Geometry: see drawing. Coordinates: mm, zero at the bounding-box minimum. Coordinates: 2 decimals unless noted, no trailing zeros. Loops run counter-clockwise (first coordinate to the right, second up) from the corner with the lowest first, then second, coordinate; pieces in that order, holes last.
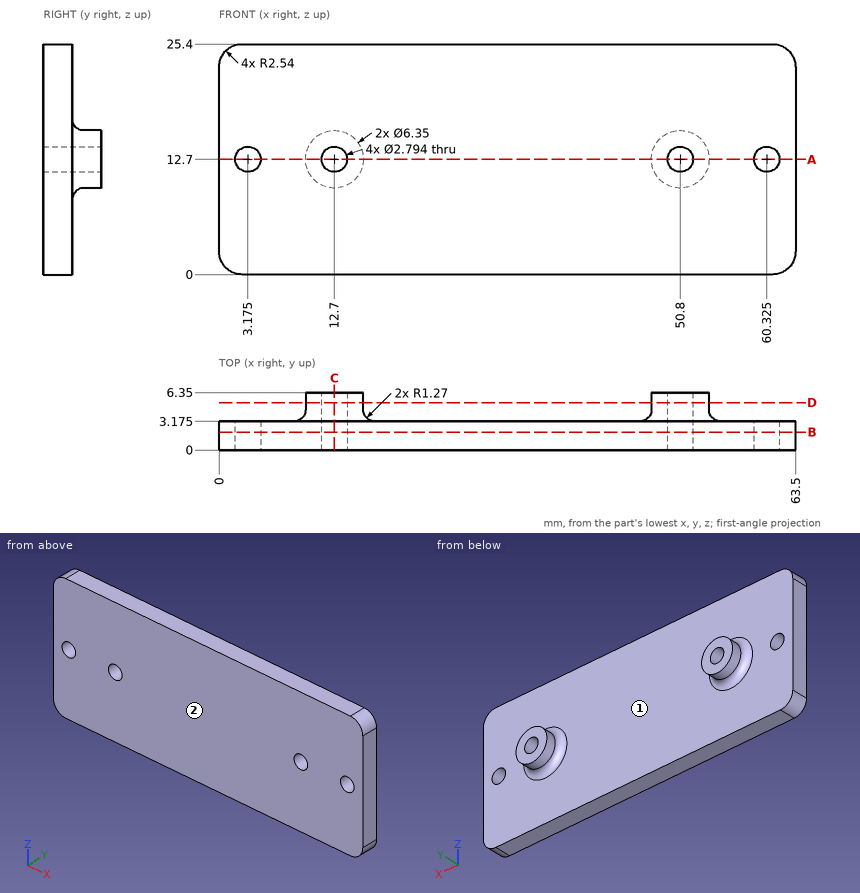
Item 1: Section query C-C (x = 12.7). Output: boundary loops of the cut face in (y, z) (3 decimals), then the cut area to 3 significant figures.
Result:
outline: (0, 0) - (3.175, 0) - (3.175, 8.255) arc R1.27 cw to (4.445, 9.525) - (6.35, 9.525) - (6.35, 11.303) - (0, 11.303) - close; (0, 14.097) - (6.35, 14.097) - (6.35, 15.875) - (4.445, 15.875) arc R1.27 cw to (3.175, 17.145) - (3.175, 25.4) - (0, 25.4) - close
area: 83.8 mm2
Item 2: Line query: L1, parallel to Z at x = 51, y = 1; L2, parallel to Z at x = 50.8, y = 5 (3 decimals); L3, parallel to Y at x = 31, z = 12 (3 decimals). Output: solid intervals per line, ascending.
Result:
L1: z = 0 to 11.32, 14.08 to 25.4
L2: z = 9.525 to 11.303, 14.097 to 15.875
L3: y = 0 to 3.175
Item 3: Mould query, pull axis X, two halves, no side actions, for the marked faces 1 and 2. Classes: +X half, -X half, draft (parallel to the pull), parting line (faces both ways), or undercut.
Result:
face 1: undercut
face 2: draft
Item 4: Section query A-A (z = 12.7). Count the separate pieces of the cut face and the enclosed holes in it, then the cut area to 3 significant figures.
Result:
separate pieces: 5
enclosed holes: 0
area: 190 mm2
Item 5: Section query D-D (y = 5.25). Output: boundary loops of the cut face in (x, z) (3 decimals), then the cut area to 3 significant figures.
Result:
outline: circle Ø6.35 at (12.7, 12.7); circle Ø6.35 at (50.8, 12.7); hole circle Ø2.794 at (12.7, 12.7); hole circle Ø2.794 at (50.8, 12.7)
area: 51.1 mm2
Item 6: Section query B-B (y = 2). Output: boundary loops of the cut face in (x, z) (3 decimals), then the cut area to 3 significant figures.
Result:
outline: (0, 2.54) arc R2.54 ccw to (2.54, 0) - (60.96, 0) arc R2.54 ccw to (63.5, 2.54) - (63.5, 22.86) arc R2.54 ccw to (60.96, 25.4) - (2.54, 25.4) arc R2.54 ccw to (0, 22.86) - close; hole circle Ø2.794 at (3.175, 12.7); hole circle Ø2.794 at (12.7, 12.7); hole circle Ø2.794 at (50.8, 12.7); hole circle Ø2.794 at (60.325, 12.7)
area: 1,580 mm2
Item 7: Contact query for a flat-ended pin moving along its axis: P1, Ø8, axis at x = 35.5, z = 20.5, coming from the +Y side (3 decimals). Output: stop coordinate, or through.
Result:
P1: stops at y = 3.175
